Can you work these out from the model? Positions are in its coordinate system, mm. A direction names the side the tool comes from. Coordinates: 2 decimals unless noted, no trailing zeros. Write each loop counter-clockwise with the first axis right and the second up, starting at its lowest first coordinate (ties: lowest second). Pieces come first, ordered by that corner, then holes. Notation, with made-up numbers: (33.25, 55.25) -> (72.25, 55.25) arc R30 ccw to (72.25, 87.25) -> close; hole circle Ø1 at (53.25, -2). An arc over 180 degrees is marked (long way). Use one line per item in the form item = value.
```python
from build123d import *

# Parameters (mm, degrees)
F0_R           = 9
F1_DEPTH       = 15
F1_DEPTH_BACK  = 15
F3_D           = 3
F3_DEPTH       = 20
F3_CSINK_D     = 6
F3_CSINK_ANGLE = 90
F4_R           = 3
F5_DEPTH       = 10
F6_SIZE        = 4


with BuildPart() as f1:
    # F0 (on Front) → F1 (new body, two sides)
    with BuildSketch(Plane.XZ) as f1_sk:
        Polygon((0, 10), (0, 0), (50, 0), (50, 10), (40, 10), (40, 75), (10, 75), (10, 10), align=None)
        with Locations((25, 55)):
            Circle(F0_R, mode=Mode.SUBTRACT)
    extrude(amount=F1_DEPTH)
    extrude(f1_sk.sketch, amount=-F1_DEPTH_BACK)

    # F3
    with Locations(Plane.XY.offset(75)):
        with Locations((25, 0)):
            CounterSinkHole(F3_D / 2, F3_CSINK_D / 2, depth=F3_DEPTH, counter_sink_angle=F3_CSINK_ANGLE)

    # F4 (on face) → F5 (cut)
    with BuildSketch(Plane.XY.offset(10)):
        with Locations((5, 10)):
            Circle(F4_R)
        with Locations((5, -10)):
            Circle(F4_R)
        with Locations((45, -10)):
            Circle(F4_R)
        with Locations((45, 10)):
            Circle(F4_R)
    extrude(amount=-F5_DEPTH, mode=Mode.SUBTRACT)

    # F6
    f6_edges = [f1.edges().sort_by_distance(p)[0] for p in [
        (40, 0, 75),
        (10, 0, 75),
    ]]
    chamfer(f6_edges, length=F6_SIZE)


solid = f1.part
```
Q1. Suppose I cut it at C-C (z = 55). Write out the boundary of the cut face in (x, y), then the cut area to 3 significant figures.
Return value:
outline = (10, -15) -> (16, -15) -> (16, 15) -> (10, 15) -> close; (34, -15) -> (40, -15) -> (40, 15) -> (34, 15) -> close
area = 360 mm2
Q2. Suppose I cut it at B-B (x = 25). Write out the boundary of the cut face in (y, z).
Return value:
outline = (-15, 0) -> (15, 0) -> (15, 46) -> (-15, 46) -> close; (-15, 64) -> (-1.5, 64) -> (-1.5, 73.5) -> (-3, 75) -> (-15, 75) -> close; (1.5, 64) -> (15, 64) -> (15, 75) -> (3, 75) -> (1.5, 73.5) -> close
Q3. Thinking about a two-plate mould opening in Y: for faces 1 (the flat face through (25, 15, 30)), 2 (the cylindrical face through (5, -7, 5)), 3 (the flat face through (5, 0, 10)), which applies, released by +Y, released by -Y, zero draft, split by the parting line, or undercut?
Return value:
face_1 = released by +Y
face_2 = undercut
face_3 = zero draft
Q4. Suppose I cut it at D-D (y = 6). Write out the boundary of the cut face in (x, z), then the cut area to 3 significant figures.
Return value:
outline = (0, 0) -> (50, 0) -> (50, 10) -> (40, 10) -> (40, 71) -> (36, 75) -> (14, 75) -> (10, 71) -> (10, 10) -> (0, 10) -> close; hole circle Ø18 at (25, 55)
area = 2,180 mm2
Q5. Will these pins go through, and if not, where does the flat tip stop? pin 1 (9.5 mm diameter, centred on x = 5, y = -10, fed in from -Z); pin 2 (3 mm diameter, centred on x = 6, y = 1, fed in from +Z); pin 3 (15 mm diameter, centred on y = 0, z = 46.5, fed in from +X); pin 4 (15 mm diameter, centred on y = 4, z = 35.5, fed in from -X).
Return value:
pin_1 = 0
pin_2 = 10
pin_3 = 40
pin_4 = 10
Q6. For faces 4 (the cylindrical face through (42, 10, 5)), 5 (the flat face through (40, 0, 40)), 6 (the flat face through (10, 0, 41)), which set-ups out of +Z, -Z, +X, -X, +Y, -Y let a thin tool reach every point of the face, with its end or its side?
Return value:
face_4 = +Z, -Z
face_5 = +Z, +X, +Y, -Y
face_6 = +Z, -X, +Y, -Y
Q7. Suppose I cut it at A-A (y = 10). Write out the boundary of the cut face in (x, z).
Return value:
outline = (0, 0) -> (2, 0) -> (2, 10) -> (0, 10) -> close; (8, 0) -> (42, 0) -> (42, 10) -> (40, 10) -> (40, 71) -> (36, 75) -> (14, 75) -> (10, 71) -> (10, 10) -> (8, 10) -> close; (48, 0) -> (50, 0) -> (50, 10) -> (48, 10) -> close; hole circle Ø18 at (25, 55)
Q8. If I drill on line 1 (Y direction, x = 5, z = 7); line 2 (Z direction, x = 47, y = 0); line 3 (Y direction, x = 25, z = 70.5), over which ranges is the centre line in solid material (lowest first)? Write a range as from..to.
Return value:
line_1 = -15..-13, -7..7, 13..15
line_2 = 0..10
line_3 = -15..-1.5, 1.5..15
